The listing builds one solid part. Answer for the finished solid, in the listing's coordinates (mm). A direction names the side the tool comes from. Give positions to 0.01 mm unless a question says otherwise; leave off trailing zeros. Loops run counter-clockwise (first coordinate to the right, second up) from the corner with the lowest first, then second, coordinate; pieces in that order, holes last. Notation, with made-up numbers: M 34,49.5 L 84,49.5 A37 cw 84,86.5 Z; hole C -25.5,41.25 d4. An arc over 180 degrees is marked long. One line per item, written item: value. Start each with the question number.
Q1. For faces 1 (the flat face through (-7, 1, 21)), 2 (the flat face through (7.11, 9.78, 29.94)), 3 (the flat face through (-7, 1, 18)), 4 (the flat face through (7, 1, 18)), 5 (the flat face through (0, 2, 12)), determine the directions among +Z, -Z, +X, -X, +Y, -Y from which every point of the face is accessible in a straight line to the end or side of a thin tool.
Q2. Consider L1, parallel to Z at x = 0, y = 1.4; L2, parallel to Z at x = 0, y = 1.2; L3, parallel to X at y = 1.3, z = 5.7. Determine where each line is inside the solid, lowest interval first.
Q3. A cutting plane is placed at A-A, the plane x = -7.25. Determine the outline of the cut face in (y, z), and give its area (3 significant figures).
Q4. The mould has two halves that part along X. Classify faces 6 (the cylindrical face through (0.08, 0.73, 24.78)), 7 (the cylindrical face through (0.556, 1.014, 3.935)), 8 (the cylindrical face through (0.08, 1.01, 18.75)), 9 (the flat face through (-5.75, 1, 12)): +X half, -X half, draft (parallel to the pull), parting line (faces both ways), or undercut.
Q5. A cutting plane is placed at C-C, the plane x = 0.75. Determine the outline of the cut face in (y, z).
Q6. A cutting plane is placed at B-B, the plane z = 16.9. Determine the outline of the cut face in (x, y), and give its area (3 significant figures).
Q7. Flat-ended cylindrical pins translate along their axes: pin 1 (1 mm diameter, centred on x = 4.5, y = 4, fed in from +Z); pin 2 (1 mm diameter, centred on x = 3.5, y = 5, fed in from -Z); pin 3 (1.5 mm diameter, centred on x = 3, z = 29, fed in from -Y); pin 4 (3 mm diameter, centred on x = 0, z = 16.9, fed in from -Y). Find the tip coordinate at first contact, or state that the pin passes through.
Q8. A cutting plane is placed at D-D, the plane z = 9. Determine the outline of the cut face in (x, y), and give its area (3 significant figures).
from build123d import *

# Parameters (mm, degrees)
T_LE_DE_BASE_PLI_E1_DEPTH = 5.75
ESQUISSE6_W               = 2
ESQUISSE6_H               = 3
PATTE1_DEPTH              = 2
ESQUISSE9_W               = 2.75
ESQUISSE9_H               = 3.5
PATTE2_DEPTH              = 2
ESQUISSE12_R              = 1.85
ENL_V_MAT_EXTRU_1_DEPTH   = 10
CONG_1_R                  = 5.75


# Sheet-metal steps are written as plain solids
with BuildPart() as part:
    # Esquisse1 → Tôle de base pliée1 (new body)
    with BuildSketch(Plane(origin=(0, 0, 0), x_dir=(0, 0, -1), z_dir=(1, 0, 0))):
        with BuildLine():
            Line((0, 0), (-22.919645957, 0))
            ThreePointArc((-22.919645957, 0), (-24.797039301, 0.745526473), (-25.651523607, 2.575901315))
            Line((-25.651523607, 2.575901315), (-25.961852844, 7.85149835))
            ThreePointArc((-25.961852844, 7.85149835), (-26.174296323, 8.327060048), (-26.648183844, 8.543212256))
            Line((-26.648183844, 8.543212256), (-33.5, 9))
            Line((-33.5, 9), (-33.366961979, 10.995570316))
            Line((-33.366961979, 10.995570316), (-26.515145823, 10.538782572))
            ThreePointArc((-26.515145823, 10.538782572), (-24.754569405, 9.735738676), (-23.965304098, 7.968942394))
            Line((-23.965304098, 7.968942394), (-23.65497486, 2.693345359))
            ThreePointArc((-23.65497486, 2.693345359), (-23.424976637, 2.200670467), (-22.919645957, 2))
            Line((-22.919645957, 2), (0, 2))
            Line((0, 2), (0, 0))
        make_face()
    extrude(amount=T_LE_DE_BASE_PLI_E1_DEPTH)

    # Esquisse6 → Patte1 (add)
    with BuildSketch(Plane(origin=(0, 2, 0), x_dir=(1, 0, 0), z_dir=(0, 1, 0))):
        with Locations((6.75, -19.5)):
            Rectangle(ESQUISSE6_W, ESQUISSE6_H)
    extrude(amount=-PATTE1_DEPTH)

    # Esquisse9 → Patte2 (add)
    with BuildSketch(Plane(origin=(0, 8.732295979, -0.582153065), x_dir=(1, 0, 0), z_dir=(0, 0.997785157856609, -0.06651901052377376))):
        with Locations((7.125, -32.274473883)):
            Rectangle(ESQUISSE9_W, ESQUISSE9_H)
    extrude(amount=-PATTE2_DEPTH)

    # Esquisse12 → Enlèv. mat.-Extru.1 (cut)
    with BuildSketch(Plane(origin=(0, 2, 0), x_dir=(1, 0, 0), z_dir=(0, 1, 0))):
        with Locations((0, -5.7)):
            Circle(ESQUISSE12_R)
        with Locations((0, -16.9)):
            Circle(ESQUISSE12_R)
    extrude(amount=-ENL_V_MAT_EXTRU_1_DEPTH, mode=Mode.SUBTRACT)

    # Congé1
    cong_1_edges = [part.edges().sort_by_distance(p)[0] for p in [
        (5.75, 1, 0),
    ]]
    fillet(cong_1_edges, radius=CONG_1_R - 0.0001)  # a hair under: the kernel refuses the full size

    # Symétrie1: part across plane


with BuildPart() as part_1:
    add(part.part)
    add(part.part.mirror(Plane(origin=(0, 2.693345359, 23.65497486), x_dir=(0, 0, 1), z_dir=(-1, 0, 0))))


solid = part_1.part
Answer block:
1. face 1: +Z, -X, +Y, -Y
1. face 2: -Z, +X, -Y
1. face 3: -Z, -X, +Y, -Y
1. face 4: -Z, +X, +Y, -Y
1. face 5: -Z, +X, -X, +Y
2. L1: 0 to 3.85, 7.55 to 15.05, 18.75 to 25.31
2. L2: 0 to 3.85, 7.55 to 15.05, 18.75 to 25.18
2. L3: -5.75 to -1.85, 1.85 to 5.75
3. outline: M 0,18 L 2,18 L 2,21 L 0,21 Z; M 8.77,30.01 L 10.76,29.87 L 11,33.37 L 9,33.5 Z
3. area: 13.0 mm^2
4. face 6: draft
4. face 7: undercut
4. face 8: undercut
4. face 9: -X half
5. outline: M 0,0.05 L 2,0.05 L 2,4.01 L 0,4.01 Z; M 0,7.39 L 2,7.39 L 2,15.21 L 0,15.21 Z; M 0,18.59 L 2,18.59 L 2,22.92 A0.74 cw 2.69,23.65 L 7.97,23.97 A2.74 ccw 10.54,26.52 L 11,33.37 L 9,33.5 L 8.54,26.65 A0.74 cw 7.85,25.96 L 2.58,25.65 A2.74 ccw 0,22.92 Z
6. outline: M -5.75,0 L -1.85,0 L -1.85,2 L -5.75,2 Z; M 1.85,0 L 5.75,0 L 5.75,2 L 1.85,2 Z
6. area: 15.6 mm^2
7. pin 1: z = 25.76
7. pin 2: z = 23.76
7. pin 3: y = 8.65
7. pin 4: through
8. outline: M -5.75,0 L 5.75,0 L 5.75,2 L -5.75,2 Z
8. area: 23.0 mm^2
